from build123d import *

# Parameters (mm, degrees)
SKETCH1_W           = 128
SKETCH1_H           = 101.6
BOSS_EXTRUDE1_DEPTH = 1
CUT_EXTRUDE1_DEPTH  = 1
SKETCH3_R           = 14.3
SKETCH3_R_2         = 7.5
CUT_EXTRUDE2_DEPTH  = 1


with BuildPart() as part:
    # Sketch1 → Boss-Extrude1 (new body)
    with BuildSketch(Plane(origin=(0, 0, 0), x_dir=(1, 0, 0), z_dir=(0, 1, 0))):
        Rectangle(SKETCH1_W, SKETCH1_H)
    extrude(amount=BOSS_EXTRUDE1_DEPTH)

    # Sketch2 → Cut-Extrude1 (cut)
    with BuildSketch(Plane(origin=(0, 1, 0), x_dir=(1, 0, 0), z_dir=(0, 1, 0))):
        with BuildLine():
            Line((-64, -50.8), (-64, -19.42235648))
            ThreePointArc((-64, -19.42235648), (-54.809700991, -41.609700991), (-32.62235648, -50.8))
            Line((-32.62235648, -50.8), (-64, -50.8))
        make_face()
        with BuildLine():
            Line((47.49, -50.8), (64, -50.8))
            Line((64, -50.8), (64, -34.29))
            ThreePointArc((64, -34.29), (59.164332957, -45.964332957), (47.49, -50.8))
        make_face()
        with BuildLine():
            Line((-64, 30.923649501), (-64, 50.8))
            Line((-64, 50.8), (-44.123649501, 50.8))
            ThreePointArc((-44.123649501, 50.8), (-58.178351724, 44.978351724), (-64, 30.923649501))
        make_face()
        with BuildLine():
            Line((64, 20.116458758), (64, 50.8))
            Line((64, 50.8), (33.316458758, 50.8))
            ThreePointArc((33.316458758, 50.8), (55.012998841, 41.812998841), (64, 20.116458758))
        make_face()
    extrude(amount=-CUT_EXTRUDE1_DEPTH, mode=Mode.SUBTRACT)

    # Sketch3 → Cut-Extrude2 (cut)
    with BuildSketch(Plane(origin=(0, 1, 0), x_dir=(1, 0, 0), z_dir=(0, 1, 0))):
        with Locations(Location((46, -32.8, 0), (0, 0, 270))):
            Circle(SKETCH3_R)
        with Locations(Location((7.3, -26, 0), (0, 0, 270))):
            Circle(SKETCH3_R_2)
        with Locations(Location((-28.7, 15.2, 0), (0, 0, 270))):
            Circle(SKETCH3_R_2)
        with Locations(Location((28.4, 15.2, 0), (0, 0, 270))):
            Circle(SKETCH3_R_2)
    extrude(amount=-CUT_EXTRUDE2_DEPTH, mode=Mode.SUBTRACT)


solid = part.part
Geometry check sheet. Reference: the model listing, model coordinates, mm. Round coordinates to 2 decimals unless told otherwise and drop trailing zeros. Loops run counter-clockwise (first coordinate to the right, second up) from the corner with the lowest first, then second, coordinate; pieces in that order, holes last. Notation, with made-up numbers: (-20.5, -31) - (-4.5, -31) arc R13 ccw to (-4.5, -27) - close; hole circle Ø4 at (3.5, 88.25). An arc over 180 degrees is marked (long way). Answer as CSV lines item,"result".
(1) Cross-section at A-A, the plane z = -15.2. Enter the section's corners in (x, y).
Output values:
outline,"(-64, 0) - (-36.2, 0) - (-36.2, 1) - (-64, 1) - close; (-21.2, 0) - (20.9, 0) - (20.9, 1) - (-21.2, 1) - close; (35.9, 0) - (64, 0) - (64, 1) - (35.9, 1) - close"
(2) Cross-section at C-C, the plane x = 7.3. Enter the section's corners in (y, z).
Output values:
outline,"(0, -50.8) - (1, -50.8) - (1, 18.5) - (0, 18.5) - close; (0, 33.5) - (1, 33.5) - (1, 50.8) - (0, 50.8) - close"
(3) Release check for a two-part mould opening along Z. For faces 1 (the face through (-31.57, 0.51, -8.27)), 2 (the face through (50.3, 0.51, 46.44)), 3 (the face through (54.773, 0.507, -42.05)), 4 (the face through (59.29, 0.51, 45.84)) record: released by +Z, released by -Z, zero draft, split by the parting line, or undercut.
Output values:
face 1,"undercut"
face 2,"undercut"
face 3,"released by -Z"
face 4,"released by +Z"
(4) Material ranges on line 1 along X through (y, z) = (0.4, -15.2); line 2 along X through (y, z) = (0.2, 26); line 3 along Z through (x, y) = (28.5, 0.75), recorded low to high.
Output values:
line 1,"x = -64 to -36.2, -21.2 to 20.9, 35.9 to 64"
line 2,"x = -63.3 to -0.2, 14.8 to 33.42, 58.58 to 64"
line 3,"z = -50.8 to -22.7, -7.7 to 50.8"
(5) Cross-section at D-D, the plane z = 24. Enter the section's corners in (x, y), and give its area (3 significant figures).
Output values:
outline,"(-63.66, 0) - (0.07, 0) - (0.07, 1) - (-63.66, 1) - close; (14.53, 0) - (34.73, 0) - (34.73, 1) - (14.53, 1) - close; (57.27, 0) - (64, 0) - (64, 1) - (57.27, 1) - close"
area,"90.7 mm²"
(6) Cross-section at B-B, the plane y = 0.55. Enter the section's corners in (x, z).
Output values:
outline,"(-64, -30.92) arc R19.88 ccw to (-44.12, -50.8) - (33.32, -50.8) arc R30.68 ccw to (64, -20.12) - (64, 34.29) arc R16.51 ccw to (47.49, 50.8) - (-32.62, 50.8) arc R31.38 ccw to (-64, 19.42) - close; hole circle Ø15 at (-28.7, -15.2); hole circle Ø15 at (7.3, 26); hole circle Ø15 at (28.4, -15.2); hole circle Ø28.6 at (46, 32.8)"
